```python
from build123d import *

# Parameters (mm, degrees)
SKETCH1_R           = 6.4516
BOSS_EXTRUDE1_DEPTH = 66.04


with BuildPart() as part:
    # Sketch1 → Boss-Extrude1 (new body)
    with BuildSketch(Plane(origin=(0, 0, 0), x_dir=(1, 0, 0), z_dir=(0, 1, 0))):
        with Locations(Location((0, 0, 0), (0, 0, 270))):
            Circle(SKETCH1_R)
    extrude(amount=BOSS_EXTRUDE1_DEPTH)

    # Sketch2 → Revolve1 (revolve)
    with BuildSketch(Plane(origin=(0, 0, 0), x_dir=(0, 0, -1), z_dir=(1, 0, 0)), mode=Mode.PRIVATE) as revolve1_sk:
        Polygon((0, 66.04), (0, 76.54), (-1.5, 76.54), (-1.5, 68.04), (-2.5, 68.04), (-2.5, 67.04), (-3, 67.04), (-3, 66.04), align=None)
    revolve(revolve1_sk.sketch.rotate(Axis((0, 66.04, 0), (0, 1, 0)), 180), axis=Axis((0, 66.04, 0), (0, 1, 0)))


solid = part.part
```
The listing builds one solid part. Answer for the finished solid, in the listing's coordinates (mm). A direction names the side the tool comes from. Give positions to 0.01 mm unless a question says otherwise; leave off trailing zeros. Write each loop counter-clockwise with the first axis right and the second up, starting at its lowest first coordinate (ties: lowest second). Pieces come first, ordered by that corner, then holes. Notation, with made-up numbers: M 63,27 L 71,27 A18 cw 71,36 Z; hole C -37.75,-33.5 d2. An arc over 180 degrees is marked long. Write each question's results on one line, items separated by ' | '.
Q1. Consider L1, parallel to Y at x = 3.75, z = -0.25; L2, parallel to X at y = 49, z = 5.25; L3, parallel to Z at x = -4, y = 20.5. Determine where each line is inside the solid, lowest interval first. Write a range as from..to.
Output values:
L1: 0..66.04 | L2: -3.75..3.75 | L3: -5.06..5.06
Q2. For a pull along Y with two mould halves and no side action, classify faces 1 (the flat face through (0, 0, 0)), 2 (the cylindrical face through (-0.45, 72.23, -1.43)), 3 (the flat face through (0, 76.54, 0)) as released by +Y, released by -Y, zero draft, split by the parting line, or undercut.
Output values:
face 1: released by -Y | face 2: zero draft | face 3: released by +Y
Q3. A tool of negligible diameter and unlimited length cuts with its end or side. For faces 4 (the cylindrical face through (1.938, 32.558, 6.154)), 5 (the cylindrical face through (-0.1, 67.5, 2.5)), from which of +Z, -Z, +X, -X, +Y, -Y can it reach the whole face along a straight path? Write none if from no direction.
Output values:
face 4: +Y, -Y | face 5: +Y
Q4. Flat-ended cylindrical pins translate along their axes: P1, Ø2, axis at x = -2.5, y = 59, coming from the -Z side; P2, Ø3, axis at x = 5, y = 48.5, coming from the +Z side; P3, Ø6, axis at x = 4, y = 28.5, coming from the +Z side. Find the tip coordinate at first contact, or state that the pin passes through.
Output values:
P1: z = -6.27 | P2: z = 5.42 | P3: z = 6.37
Q5. Section A-A, the plane z = 0 is taken. Write down the section's boundary in (x, y), then the cut area to 3 significant figures.
Output values:
outline: M -6.45,0 L 6.45,0 L 6.45,66.04 L 3,66.04 L 3,67.04 L 2.5,67.04 L 2.5,68.04 L 1.5,68.04 L 1.5,76.54 L -1.5,76.54 L -1.5,68.04 L -2.5,68.04 L -2.5,67.04 L -3,67.04 L -3,66.04 L -6.45,66.04 Z | area: 889 mm2
Q6. Section B-B, the plane x = 0 is taken. Write down the section's boundary in (y, z), then the cut area to 3 significant figures.
Output values:
outline: M 0,-6.45 L 66.04,-6.45 L 66.04,-3 L 67.04,-3 L 67.04,-2.5 L 68.04,-2.5 L 68.04,-1.5 L 76.54,-1.5 L 76.54,1.5 L 68.04,1.5 L 68.04,2.5 L 67.04,2.5 L 67.04,3 L 66.04,3 L 66.04,6.45 L 0,6.45 Z | area: 889 mm2
Q7. Section D-D, the plane x = -5 is taken. Write down the section's boundary in (y, z).
Output values:
outline: M 0,-4.08 L 66.04,-4.08 L 66.04,4.08 L 0,4.08 Z
Q8. Section C-C, the plane y = 23 is taken. Write down the section's boundary in (x, z).
Output values:
outline: C 0,0 d12.9
